```python
from build123d import *

# Parameters (mm, degrees)
F0_R     = 47.600257
F1_DEPTH = 120
F2_R     = 28.82737
F3_DEPTH = 120.001
F4_R     = 124.230841
F4_R_2   = 28.82737
F5_DEPTH = 60
F8_R     = 53.98765
F9_DEPTH = 120


with BuildPart() as f1:
    # F0 (on Front) → F1 (new body)
    with BuildSketch(Plane.XZ):
        Circle(F0_R)
    extrude(amount=F1_DEPTH)

    # F2 (on face) → F3 (cut, through all)
    with BuildSketch(Plane.XZ.offset(120)):
        Circle(F2_R)
    extrude(amount=-F3_DEPTH, mode=Mode.SUBTRACT)

    # F2 (on face) + F4 (on face) → F5 (join)
    with BuildSketch(Plane.XZ.offset(120)):
        Circle(F2_R)
    with BuildSketch(Plane.XZ.offset(120)):
        Circle(F4_R)
        Circle(F4_R_2, mode=Mode.SUBTRACT)
    extrude(amount=F5_DEPTH)

    # F8 (on face) → F9 (join)
    with BuildSketch(Plane.XZ.offset(180)):
        Circle(F8_R)
    extrude(amount=F9_DEPTH)


solid = f1.part
```
CAD build for the part. Positions are in the model's coordinates, mm. A direction names the side the tool comes from. Coordinates: 2 decimals unless noted, no trailing zeros. Order: outer loops, then holes, each group sorted by start corner. A loop starts at its lowest first (then second) coordinate and runs counter-clockwise, first axis right, second up. Notation, with made-up numbers: M 44,50.5 L 93,50.5 A17 ccw 93,66.5 Z; hole C 14,23 d7. An arc over 180 degrees is marked long. Answer as CSV lines item,"result".
1) 3-axis set-ups, long thin cutter, end or side, ignore diameter. For faces 4 (the cylindrical face through (-3.753, -60.84, 28.582)), 5 (the cylindrical face through (57.325, -149.58, -110.214)), 6 (the flat face through (26, -180, -53)): which of +Z, -Z, +X, -X, +Y, -Y reach the whole face in a straight line?
Verdict:
face 4,"+Y"
face 5,"+Y, -Y"
face 6,"-Y"
2) Drill centre lines: L1, parallel to Z at x = 0, y = -60; L2, parallel to Y at x = -91, z = 32.5; L3, parallel to Z at x = 1, y = -128.5. Where is each one in solid material? Low to high. Write a range as from..to.
Verdict:
L1,"-47.6..-28.83, 28.83..47.6"
L2,"-180..-120"
L3,"-124.23..124.23"
3) Flat gauge pins, fed straight in: P1, Ø10, axis at x = -23.5, y = -153, coming from the +Z side; P2, Ø10, axis at y = -123, z = -40, coming from the +X side; P3, Ø10, axis at y = -163, z = -89, coming from the +X side. Where does each tip first touch, or does it go through?
Verdict:
P1,"z = 122.85"
P2,"x = 119.2"
P3,"x = 91.53"
4) Mould opens along X. For faces 1 (the flat face through (-2, -120, -53)), 2 (the flat face through (0, -120, 0)), 3 (the cylindrical face through (29.023, -239.16, 45.523)) say: released by +X, released by -X, zero draft, split by the parting line, or undercut.
Verdict:
face 1,"zero draft"
face 2,"undercut"
face 3,"split by the parting line"
5) Cut at B-B (z = 0). List the corners of the cut face in (x, y), then the cut area to 3 significant figures.
Verdict:
outline,"M -124.23,-180 L -53.99,-180 L -53.99,-300 L 53.99,-300 L 53.99,-180 L 124.23,-180 L 124.23,-120 L 47.6,-120 L 47.6,0 L 28.83,0 L 28.83,-120 L -28.83,-120 L -28.83,0 L -47.6,0 L -47.6,-120 L -124.23,-120 Z"
area,"32,400 mm2"
6) Cut at C-C (y = -84). List the corners of the cut face in (x, z), then the cut area to 3 significant figures.
Verdict:
outline,"C 0,0 d95.2; hole C 0,0 d57.65"
area,"4,510 mm2"
7) Cut at A-A (x = 0). List the corners of the cut face in (y, z).
Verdict:
outline,"M -300,-53.99 L -180,-53.99 L -180,-124.23 L -120,-124.23 L -120,-47.6 L 0,-47.6 L 0,-28.83 L -120,-28.83 L -120,28.83 L 0,28.83 L 0,47.6 L -120,47.6 L -120,124.23 L -180,124.23 L -180,53.99 L -300,53.99 Z"
8) Cut at D-D (y = -130). List the corners of the cut face in (x, z), then the cut area to 3 significant figures.
Verdict:
outline,"C 0,0 d248.46"
area,"48,500 mm2"
